The drawing under review shows one solid part. Ordinate dimensions are in mm from its lowest x, y, z. Round coordinates to 2 decimals unless told otherwise and drop trailing zeros. Write each loop counter-clockwise with the first axis right and the second up, starting at its lowest first coordinate (ties: lowest second). Pieces come first, ordered by that corner, then holes. Notation, with made-up numbers: (18.25, -18.5) -> (24.25, -18.5) arc R20 ccw to (24.25, 13.5) -> close; hole circle Ø4 at (4.25, 33.25). An arc over 180 degrees is marked (long way). Write item = value, one per line. Start each with the question number.
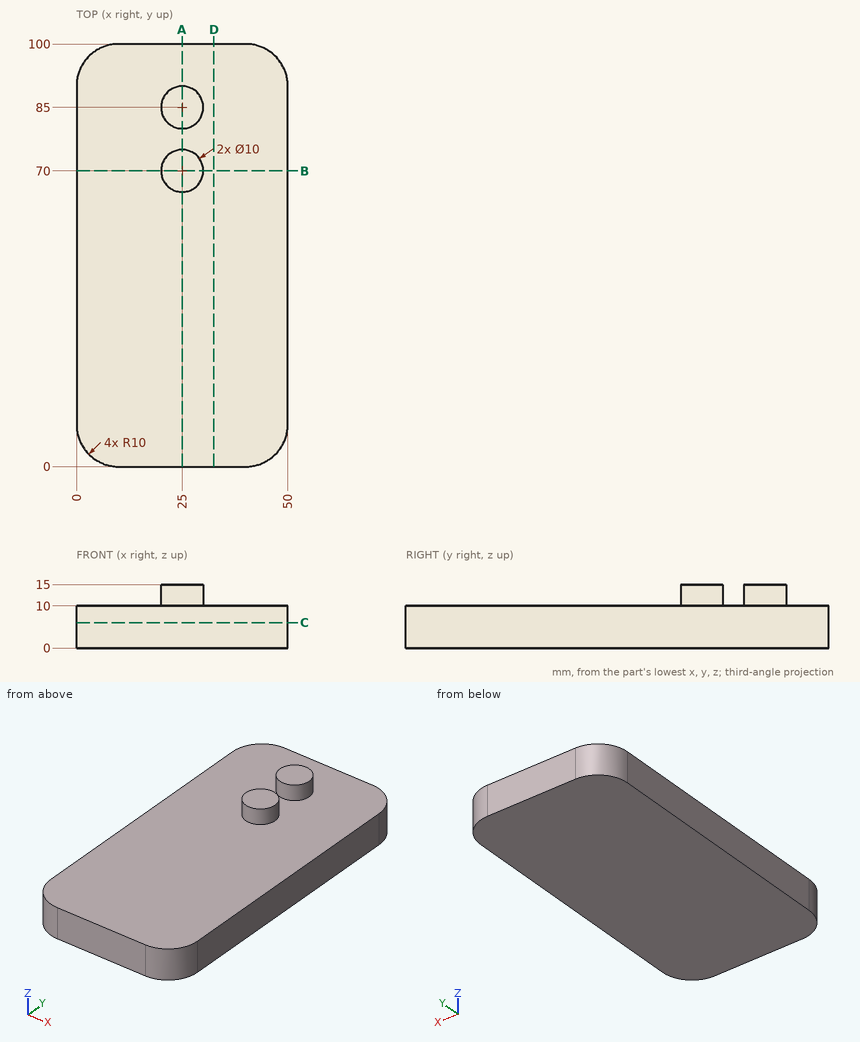
1. Clearance check with flat-ended pins moving along their axes: pin 1 Ø4 at (x, y) = (39.5, 72) entering from -Z; pin 2 Ø1.5 at (x, z) = (9, 8) entering from -Y; pin 3 Ø4 at (x, y) = (33, 80.5) entering from +Z. State where each tip first meets the part, or that it passes through.
2. Consider section C-C, the plane z = 6. Give the boundary of the cut face in (x, y), then the cut area to 3 significant figures.
3. Consider section A-A, the plane x = 25. Give the boundary of the cut face in (y, z).
4. Consider section D-D, the plane x = 32.5. Give the boundary of the cut face in (y, z).
5. Wall thickness on L1, parallel to Z at x = 8.5, y = 90.5; L2, parallel to X at y = 7, z = 1.5; L3, parallel to X at y = 80.5, z = 10.25: over which ranges is each line inside the solid? List them lowest first. Write a range as from..to.
6. Consider section B-B, the plane y = 70. Give the boundary of the cut face in (x, z), then the cut area to 3 significant figures.
Outcome:
q1.pin_1 = 0
q1.pin_2 = 0
q1.pin_3 = 10
q2.outline = (0, 10) arc R10 ccw to (10, 0) -> (40, 0) arc R10 ccw to (50, 10) -> (50, 90) arc R10 ccw to (40, 100) -> (10, 100) arc R10 ccw to (0, 90) -> close
q2.area = 4,910 mm2
q3.outline = (0, 0) -> (100, 0) -> (100, 10) -> (90, 10) -> (90, 15) -> (80, 15) -> (80, 10) -> (75, 10) -> (75, 15) -> (65, 15) -> (65, 10) -> (0, 10) -> close
q4.outline = (0, 0) -> (100, 0) -> (100, 10) -> (0, 10) -> close
q5.L1 = 0..10
q5.L2 = 0.46..49.54
q5.L3 = 22.82..27.18
q6.outline = (0, 0) -> (50, 0) -> (50, 10) -> (30, 10) -> (30, 15) -> (20, 15) -> (20, 10) -> (0, 10) -> close
q6.area = 550 mm2
